from build123d import *

# Parameters (mm, degrees)
SKETCH1_W                = 98
SKETCH1_H                = 82
BOSS_EXTRUDE1_DEPTH      = 12
CUT_EXTRUDE1_REACH       = 67.008
SKETCH4_W                = 32
SKETCH4_H                = 12
F_5_0_5_DIAMETER_HOLE2_D = 5
F_5_0_5_DIAMETER_HOLE3_D = 5
CUT_EXTRUDE3_DEPTH       = 8
CUT_EXTRUDE4_DEPTH       = 6.5
F_5_0_5_DIAMETER_HOLE1_D = 5
CUT_EXTRUDE2_REACH       = 67.008


# Read off the part's stored shape, not the designer's step: Cut-Extrude3
with BuildPart() as part:
    # Sketch1 → Boss-Extrude1 (new body)
    with BuildSketch(Plane.XY):
        Rectangle(SKETCH1_W, SKETCH1_H)
    extrude(amount=BOSS_EXTRUDE1_DEPTH)

    # Sketch4 → Cut-Extrude1 (cut, up to next)
    with BuildSketch(Plane.XY.offset(12), mode=Mode.PRIVATE) as cut_extrude1_sk1:
        with Locations((-33, 35)):
            Rectangle(SKETCH4_W, SKETCH4_H)
    cut_extrude1_tool1 = extrude(cut_extrude1_sk1.sketch, amount=-CUT_EXTRUDE1_REACH, mode=Mode.PRIVATE) & part.part
    cut_extrude1 = cut_extrude1_tool1.solids().sort_by_distance((-33, 35, 12))[0]
    add(cut_extrude1, mode=Mode.SUBTRACT)

    # Mirror2: Cut-Extrude1 across plane
    add(cut_extrude1.mirror(Plane(origin=(0, 0, 0), x_dir=(0, 0, 1), z_dir=(1, 0, 0))), mode=Mode.SUBTRACT)

    # Ø5.0 (5) Diameter Hole2 (through all)
    with Locations(Plane.XY.offset(12)):
        with Locations((-12.75, 19), (-12.75, -31)):
            f_5_0_5_diameter_hole2 = Hole(F_5_0_5_DIAMETER_HOLE2_D / 2)

    # Ø5.0 (5) Diameter Hole3 (through all)
    with Locations(Plane.XY.offset(12)):
        with Locations((-43.25, 19), (-43.25, -31)):
            f_5_0_5_diameter_hole3 = Hole(F_5_0_5_DIAMETER_HOLE3_D / 2)

    # Cut-Extrude3 outline → Cut-Extrude3 (cut)
    with BuildSketch(Plane.XY):
        with BuildLine():
            ThreePointArc((32, 15), (34, 17), (32, 19))
            Line((32, 19), (24, 19))
            ThreePointArc((24, 19), (22, 17), (24, 15))
            Line((24, 15), (32, 15))
        make_face()
    cut_extrude3 = extrude(amount=CUT_EXTRUDE3_DEPTH, mode=Mode.SUBTRACT)

    # Sketch20 → Cut-Extrude4 (cut)
    with BuildSketch(Plane(origin=(39.292468455, 97.580435701, 0), x_dir=(-1, 0, 0), z_dir=(0, 0, -1))):
        with BuildLine():
            Line((13.792468455, -19.569462754), (13.792468455, -85.580435701))
            ThreePointArc((13.792468455, -85.580435701), (11.292468455, -88.080435701), (8.792468455, -85.580435701))
            Line((8.792468455, -85.580435701), (8.792468455, -19.569462754))
            ThreePointArc((8.792468455, -19.569462754), (11.292468455, -17.069462754), (13.792468455, -19.569462754))
        make_face()
    cut_extrude4 = extrude(amount=-CUT_EXTRUDE4_DEPTH, mode=Mode.SUBTRACT)

    # Mirror1: Ø5.0 (5) Diameter Hole2, Ø5.0 (5) Diameter Hole3, Cut-Extrude3, Cut-Extrude4 across plane
    add(f_5_0_5_diameter_hole2.mirror(Plane(origin=(0, 0, 0), x_dir=(0, 0, 1), z_dir=(1, 0, 0))), mode=Mode.SUBTRACT)
    add(f_5_0_5_diameter_hole3.mirror(Plane(origin=(0, 0, 0), x_dir=(0, 0, 1), z_dir=(1, 0, 0))), mode=Mode.SUBTRACT)
    add(cut_extrude3.mirror(Plane(origin=(0, 0, 0), x_dir=(0, 0, 1), z_dir=(1, 0, 0))), mode=Mode.SUBTRACT)
    add(cut_extrude4.mirror(Plane(origin=(0, 0, 0), x_dir=(0, 0, 1), z_dir=(1, 0, 0))), mode=Mode.SUBTRACT)

    # Ø5.0 (5) Diameter Hole1 (through all)
    with Locations(Plane.XY.offset(12)):
        with Locations((0, 33)):
            Hole(F_5_0_5_DIAMETER_HOLE1_D / 2)

    # Sketch16 → Cut-Extrude2 (cut, up to next)
    with BuildSketch(Plane.XY.offset(12), mode=Mode.PRIVATE) as cut_extrude2_sk1:
        with BuildLine():
            Line((-21, 29), (-17, 29))
            ThreePointArc((-17, 29), (-19, 27), (-21, 29))
        make_face()
    cut_extrude2_tool1 = extrude(cut_extrude2_sk1.sketch, amount=-CUT_EXTRUDE2_REACH, mode=Mode.PRIVATE) & part.part
    # Sketch16 → Cut-Extrude2 (cut, up to next)
    with BuildSketch(Plane.XY.offset(12), mode=Mode.PRIVATE) as cut_extrude2_sk2:
        with BuildLine():
            Line((17, 29), (21, 29))
            ThreePointArc((21, 29), (19, 27), (17, 29))
        make_face()
    cut_extrude2_tool2 = extrude(cut_extrude2_sk2.sketch, amount=-CUT_EXTRUDE2_REACH, mode=Mode.PRIVATE) & part.part
    add(cut_extrude2_tool1.solids().sort_by_distance((-19, 28.151174, 12))[0], mode=Mode.SUBTRACT)
    add(cut_extrude2_tool2.solids().sort_by_distance((19, 28.151174, 12))[0], mode=Mode.SUBTRACT)


solid = part.part
The listing builds one solid part. Answer for the finished solid, in the listing's coordinates (mm). A direction names the side the tool comes from. Give positions to 0.01 mm unless a question says otherwise; leave off trailing zeros. Write each loop counter-clockwise with the first axis right and the second up, starting at its lowest first coordinate (ties: lowest second). Pieces come first, ordered by that corner, then holes.
Item 1: Which of the six approach directions +Z, -Z, +X, -X, +Y, -Y give full straight-line access (tool end or side, diameter ignored) to faces 5 (the cylindrical face through (34, 17, 4)), 6 (the cylindrical face through (-27.9, 9.5, 3.2)), 7 (the flat face through (-1, -41, 6))?
Item 2: Section D-D, the plane x = 0 is taken. Write down the section's boundary in (y, z), plus the area to 3 significant figures.
Item 3: Determine the mould class of faces 1 (the flat face through (-30.5, 24, 3)), 2 (the flat face through (0, 41, 6)), 3 (the flat face through (17, 35, 6)), 4 (the flat face through (28, 24, 6.5)) for opening direction X: released by +X, released by -X, zero draft, split by the parting line, or undercut.
Item 4: Section B-B, the plane y = 24.5 is taken. Write down the section's boundary in (x, z).
Item 5: Section C-C, the plane z = 9.75 is taken. Count the separate pieces of the cut face and the enclosed holes in it, plus the area to 3 significant figures.
Item 6: Find the intervals of material crossed by line 1 along Y through (x, z) = (-43.25, 4.5); line 2 along Y through (x, z) = (-12.75, 5.25); line 3 along Y through (x, z) = (0, 9.25), in increasing order.
Item 7: Flat-ended cylindrical pins translate along their axes: P1, Ø8, axis at x = -12.75, y = -31, coming from the -Z side; P2, Ø2.5, axis at x = -28, y = 12.5, coming from the -Z side; P3, Ø4, axis at x = -26, z = 4.5, coming from the +Y side; P4, Ø3.5, axis at y = 32.5, z = 8, coming from the +X side. Find the tip coordinate at first contact, or state that the pin passes through.
Item 8: Section A-A, the plane x = 12.75 is taken. Write down the section's boundary in (y, z), plus the area to 3 significant figures.
Completed:
1. face 5: -Z
1. face 6: -Z, +Y
1. face 7: +Z, -Z, +X, -X, -Y
2. outline: (-41, 0) - (30.5, 0) - (30.5, 12) - (-41, 12) - close; (35.5, 0) - (41, 0) - (41, 12) - (35.5, 12) - close
2. area: 924 mm2
3. face 1: undercut
3. face 2: zero draft
3. face 3: released by +X
3. face 4: undercut
4. outline: (-49, 0) - (-30.5, 0) - (-30.5, 6.5) - (-25.5, 6.5) - (-25.5, 0) - (25.5, 0) - (25.5, 6.5) - (30.5, 6.5) - (30.5, 0) - (49, 0) - (49, 12) - (-49, 12) - close
5. separate pieces: 1
5. enclosed holes: 9
5. area: 7,080 mm2
6. line 1: y = -41 to -33.5, -28.5 to 16.5, 21.5 to 29
6. line 2: y = -41 to -33.5, -28.5 to 16.5, 21.5 to 41
6. line 3: y = -41 to 30.5, 35.5 to 41
7. P1: stops at z = 0
7. P2: stops at z = 6.5
7. P3: stops at y = 29
7. P4: stops at x = 17
8. outline: (-41, 0) - (-33.5, 0) - (-33.5, 12) - (-41, 12) - close; (-28.5, 0) - (16.5, 0) - (16.5, 12) - (-28.5, 12) - close; (21.5, 0) - (41, 0) - (41, 12) - (21.5, 12) - close
8. area: 864 mm2
